```python
from build123d import *

# Parameters (mm, degrees)
F0_R     = 3
F1_DEPTH = 4
F2_R     = 1.35
F3_DEPTH = 2
F4_R     = 1.5


with BuildPart() as f1:
    # F0 (on Front) → F1 (new body)
    with BuildSketch(Plane.XZ):
        with Locations((-17.472006, 9.866998)):
            Circle(F0_R)
    extrude(amount=F1_DEPTH)

    # F2 (on face) → F3 (cut)
    with BuildSketch(Plane.XZ.offset(4)):
        with Locations((-17.472006, 9.866998)):
            Circle(F2_R)
    extrude(amount=-F3_DEPTH, mode=Mode.SUBTRACT)

    # F4
    f4_edges = [f1.edges().sort_by_distance(p)[0] for p in [
        (-20.472006, 0, 9.866998),
    ]]
    fillet(f4_edges, radius=F4_R)


solid = f1.part
```
Geometry check sheet. Reference: the model listing, model coordinates, mm. A direction names the side the tool comes from. Give positions to 0.01 mm unless a question says otherwise; leave off trailing zeros. Write each loop counter-clockwise with the first axis right and the second up, starting at its lowest first coordinate (ties: lowest second). Pieces come first, ordered by that corner, then holes. Notation, with made-up numbers: (53.5, 46.5) - (93.5, 46.5) arc R10 cw to (93.5, 54.5) - close; hole circle Ø9 at (70, 15.25). An arc over 180 degrees is marked (long way). Use a Markdown table: item, result.
Q1. Draft check along Z on faces 1 (the face through (-16, -4, 9)), 2 (the face through (-16.184, -3.014, 10.273)), 3 (the face through (-14.7, -2.73, 8.72)). Enter one of: pulls with the +Z half, pulls with the -Z half, needs draft (parallel to the pull), parting line crosses it, or undercut.
Computed:
| item | result |
|---|---|
| face 1 | needs draft |
| face 2 | undercut |
| face 3 | parting line crosses it |
Q2. Section check B-B, the plane y = -1.7. Enter the section's corners in (x, z).
Computed:
| item | result |
|---|---|
| outline | circle Ø6 at (-17.47, 9.87) |
Q3. Set-up check for faces 4 (the face through (-17, -2, 10)), 5 (the face through (-17, 0, 10)): record each of +Z, -Z, +X, -X, +Y, -Y from which the full face is reachable in a straight line by a thin tool's end or side.
Computed:
| item | result |
|---|---|
| face 4 | -Y |
| face 5 | +Z, -Z, +X, -X, +Y |
Q4. Thickness scan on L1, parallel to Z at x = -16.4, y = -2.1; L2, parallel to Z at x = -17.65, y = -3.3; L3, parallel to Y at x = -17, z = 8.7. Record the ranges inside material, lowest first. Write a range as [from, to].
Computed:
| item | result |
|---|---|
| L1 | z = [7.07, 9.05], [10.69, 12.67] |
| L2 | z = [6.87, 8.53], [11.21, 12.86] |
| L3 | y = [-2, 0] |
Q5. Go/stop test with flat-tipped pins: P1, Ø1, axis at x = -16.5, y = -3.5, coming from the +Z side; P2, Ø0.8, axis at x = -17.5, z = 9, coming from the -Y side; P3, Ø1.5, axis at y = -2, z = 8.5, coming from the +X side. Record where each tip stops, or that it passes through.
Computed:
| item | result |
|---|---|
| P1 | stops at z = 12.83 |
| P2 | stops at y = -2 |
| P3 | stops at x = -14.54 |
Q6. Section check A-A, the plane y = -3. Enter the section's corners in (x, z), then the cut area to 3 significant figures.
Computed:
| item | result |
|---|---|
| outline | circle Ø6 at (-17.47, 9.87); hole circle Ø2.7 at (-17.47, 9.87) |
| area | 22.5 mm² |
